Design review of the part shown in the three views and the two pictorial views. Dimensions are in mm from the part's minimum x, y and z. Coordinates: 2 decimals unless noted, no trailing zeros. Order: outer loops, then holes, each group sorted by start corner. A loop starts at its lowest first (then second) coordinate and runs counter-clockwise, first axis right, second up. Notation, with made-up numbers: (28, -0.75) - (61, -0.75) arc R23 cw to (61, 29.25) - close; hole circle Ø1 at (-36.5, 50). An arc over 180 degrees is marked (long way). One line per item, written item: value. Start each with the question number.
(1) Consider section A-A on x = 152.4. Write out the cut boundary in (y, z).
(2) To check wall thickness, follow line 1 along Y through (x, z) = (151.5, 1.25); line 2 along X through (y, z) = (47.5, 2.5) (1 decimal); line 3 along X through (y, z) = (66, 6.5) (1 decimal). State the ranges of each line that lie inside material, in increasing order.
(3) Consider section C-C on x = 50.8. Write out the cut boundary in (y, z) (1 decimal).
(4) Consider section B-B on y = 76.2. Write out the cut boundary in (x, z).
(5) Consider section D-D on y = 53. Write out the cut boundary in (x, z), then the cut area to 3 significant figures.
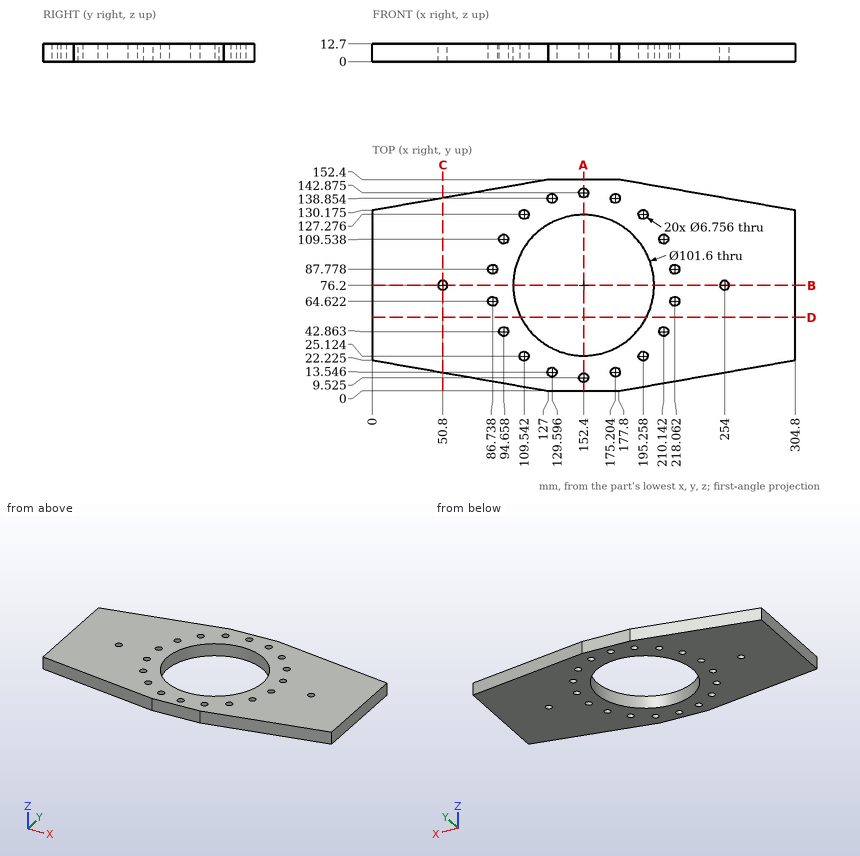
Geometry check:
1. outline: (0, 0) - (6.15, 0) - (6.15, 12.7) - (0, 12.7) - close; (12.9, 0) - (25.4, 0) - (25.4, 12.7) - (12.9, 12.7) - close; (127, 0) - (139.5, 0) - (139.5, 12.7) - (127, 12.7) - close; (146.25, 0) - (152.4, 0) - (152.4, 12.7) - (146.25, 12.7) - close
2. line 1: y = 0 to 6.27, 12.78 to 25.41, 126.99 to 139.62, 146.13 to 152.4
2. line 2: x = 0 to 110.5, 194.3 to 304.8
2. line 3: x = 0 to 83.7, 89.8 to 102.6, 202.2 to 215, 221.1 to 304.8
3. outline: (13.3, 0) - (72.8, 0) - (72.8, 12.7) - (13.3, 12.7) - close; (79.6, 0) - (139.1, 0) - (139.1, 12.7) - (79.6, 12.7) - close
4. outline: (0, 0) - (47.42, 0) - (47.42, 12.7) - (0, 12.7) - close; (54.18, 0) - (101.6, 0) - (101.6, 12.7) - (54.18, 12.7) - close; (203.2, 0) - (250.62, 0) - (250.62, 12.7) - (203.2, 12.7) - close; (257.38, 0) - (304.8, 0) - (304.8, 12.7) - (257.38, 12.7) - close
5. outline: (0, 0) - (107.21, 0) - (107.21, 12.7) - (0, 12.7) - close; (197.59, 0) - (304.8, 0) - (304.8, 12.7) - (197.59, 12.7) - close
5. area: 2,720 mm^2
